Autodesk Inventor part; units mm, degrees
ref_plane "YZ Plane" through (0, 0, 0) normal (1, 0, 0) x (0, 1, 0)
ref_plane "XZ Plane" through (0, 0, 0) normal (0, 1, 0) x (-1, 0, 0)
ref_plane "XY Plane" through (0, 0, 0) normal (0, 0, 1) x (1, 0, 0)
sketch "Sketch1" plane through (0, 0, 0) normal (0, 0, 1) x (1, 0, 0)
  line L0 (0, 0) -> (15, 0)
  line L1 (0, 0) -> (-10.6066, 10.6066)
  line L2 (0, 0) -> (15, 0) construction
  line L3 (-10.6066, 10.6066) -> (-12.3744, 8.8388)
  line L4 (15, 0) -> (15, -2.5)
  line L5 (0, 0) -> (2.3007, 5.5544) construction
  line L6 (0, 0) -> (6.0121, 0) construction
  line L7 (2.3007, 5.5544) -> (-1.6655, -4.021) construction
  line L8 (-12.3744, 8.8388) -> (-1.0355, -2.5)
  line L9 (15, -2.5) -> (-1.0355, -2.5)
  dimension "d2" = 15
  dimension "d3" = 15
  dimension "d4" = 135
  dimension "d5" = 2.5
  dimension "d6" = 2.5
  dimension "d7" = 67.5
extrude "Extrusion1" add sketch "Sketch1" along normal blind 15
sketch "Sketch2" plane through (-10.6066, 10.6066, 0) normal (0.7071, 0.7071, 0) x (-0.7071, 0.7071, 0)
  circle A0 centre (-7.5, 7.5) radius 1.75
  line L0 (-15, 15) -> (0, 15)
  line L1 (-15, 0) -> (-15, 15)
  dimension "d10" = 3.5
  dimension "d11" = 7.5
  dimension "d12" = 7.5
sketch "Sketch3" plane through (0, 0, 0) normal (0, 1, 0) x (1, 0, 0)
  circle A0 centre (7.5, -7.5) radius 1.75
  line L0 (15, 0) -> (15, -15)
  line L1 (15, 0) -> (0, 0)
  dimension "d13" = 3.5
  dimension "d14" = 7.5
  dimension "d15" = 7.5
extrude "Extrusion2" cut sketch "Sketch2" against normal blind 15
extrude "Extrusion3" cut sketch "Sketch3" against normal blind 15
fillet "Fillet1" radius 2 4 edges at (-11.4905, 9.7227, 15) (-11.4905, 9.7227, 0) (15, -1.25, 0) (15, -1.25, 15)
properties part number "45 degree inside coner bracket"
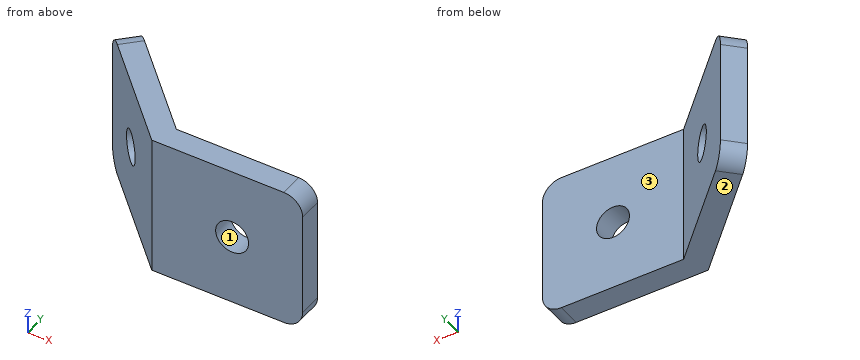
Geometry: final body of the model. Coordinates: model frame, mm. Face numbers are marked on the shaded views. Round coordinates to 2 decimals unless told otherwise and drop trailing zeros. Write each loop counter-clockwise with the first axis right and the second up, starting at its lowest first coordinate (ties: lowest second). Pieces come first, ordered by that corner, then holes.
Item 1: Section query D-D (z = 3). Return loops of the section in (x, y), plus the area to 3 significant figures.
Item 2: Pin query (flat end, axial travel): P1, Ø7.5, axis at x = 9.5, z = 6.5, coming from the +Y side; P2, Ø8, axis at x = 3.5, z = 13.5, coming from the +Y side; P3, Ø4, axis at x = -9, y = 0, coming from the +Z side; P4, Ø1.5, axis at x = -9, z = 5.5, coming from the -Y side. Return the tip coordinate at first contact, or that it passes through.
Item 3: Section query C-C (z = 7.5). Return loops of the section in (x, y).
Item 4: Section query A-A (x = 7.5). Return loops of the section in (y, z), plus the area to 4 significant figures.
Item 5: Section query B-B (y = -1). Return loops of the section in (x, z), plus the area to 3 significant figures.
Item 6: Material intervals for L1, parallel to Z at x = 7.5, y = -1.6; L2, parallel to Y at x = 10.5, z = 10.5; L3, parallel to X at y = -0.65, z = 7.5, sorted ascending.
Item 7: Mould query, pull axis Z, two halves, no side actions, for the marked faces 1, 2 and 3. Classes: +Z half, -Z half, draft (parallel to the pull), parting line (faces both ways), or undercut.
Completed:
1. outline: (-12.37, 8.84) - (-1.04, -2.5) - (15, -2.5) - (15, 0) - (0, 0) - (-10.61, 10.61) - close
1. area: 77.6 mm2
2. P1: stops at y = 0
2. P2: stops at y = 0.5
2. P3: passes through
2. P4: stops at y = 4.71
3. outline: (-12.37, 8.84) - (-8.31, 4.77) - (-6.54, 6.54) - (-10.61, 10.61) - close; (-5.83, 2.3) - (-1.04, -2.5) - (5.75, -2.5) - (5.75, 0) - (0, 0) - (-4.07, 4.07) - close; (9.25, -2.5) - (15, -2.5) - (15, 0) - (9.25, 0) - close
4. outline: (-2.5, 0) - (0, 0) - (0, 5.75) - (-2.5, 5.75) - close; (-2.5, 9.25) - (0, 9.25) - (0, 15) - (-2.5, 15) - close
4. area: 28.75 mm2
5. outline: (-2.54, 0) - (13, 0) arc R2 ccw to (15, 2) - (15, 13) arc R2 ccw to (13, 15) - (-2.54, 15) - close; hole circle Ø3.5 at (7.5, 7.5)
5. area: 252 mm2
6. L1: z = 0 to 5.75, 9.25 to 15
6. L2: y = -2.5 to 0
6. L3: x = -2.89 to 5.75, 9.25 to 15
7. face 1: undercut
7. face 2: -Z half
7. face 3: draft
